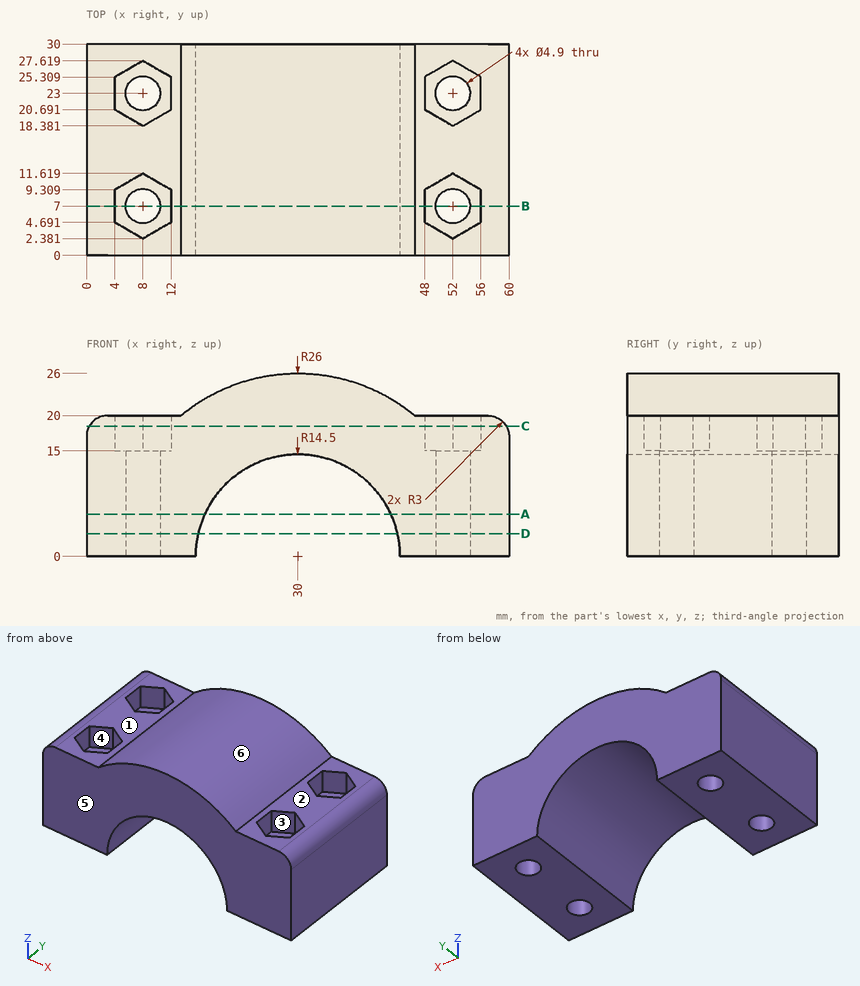
Design review of the part shown in the three views and the two pictorial views. Dimensions are in mm from the part's minimum x, y and z. A direction names the side the tool comes from. Round coordinates to 2 decimals unless told otherwise and drop trailing zeros. Write each loop counter-clockwise with the first axis right and the second up, starting at its lowest first coordinate (ties: lowest second). Pieces come first, ordered by that corner, then holes. Notation, with made-up numbers: (-15, 2) - (-8, 2) arc R28 ccw to (-8, 31) - close; hole circle Ø1 at (54.5, 51). An arc over 180 degrees is marked (long way). Answer as CSV lines item,"result". Start each with the question number.
(1) Add section A-A, the plane z = 6. State the section outline as (x, y) points.
(2) Add section D-D, the plane z = 3.25. State the section outline as (x, y) points.
(3) Mouldability with a two-part tool opening along Y and no side actions: class the marked faces 4, 5 and 6 as +Y half, -Y half, draft (parallel to the pull), parting line (faces both ways), or undercut.
(4) Add section B-B, the plane y = 7. State the section outline as (x, z) points.
(5) For pin 1 (4.5 mm diameter, centred on x = 8, y = 7, fed in from +Z); pin 2 (2 mm diameter, centred on x = 37, y = 4, fed in from +Z); pin 3 (4 mm diameter, centred on x = 7, y = 24, fed in from +Z); pin 4 (9 mm diameter, centred on x = 50, y = 7, fed in from +Z) (1 decimal), all flat-tipped, find the tip position at first contact; note any pin that passes through.
(6) For line 1 (Y direction, x = 52, z = 9.5); line 2 (X direction, y = 24.5, z = 3.5); line 3 (X direction, y = 7, z = 9.75), list the stretches that pass through material, from the lowest coordinate up.
(7) Add section C-C, the plane z = 18.5. State the section outline as (x, y) points.
(8) Machinability: for the marked faces 1, 2 and 3, which of the approach directions +Z, -Z, +X, -X, +Y, -Y give a long, thin tool a straight path to every point of the face, cutting with its end or side? Answer none if there is none.
From the geometry:
1,outline,"(0, 0) - (16.8, 0) - (16.8, 30) - (0, 30) - close; (43.2, 0) - (60, 0) - (60, 30) - (43.2, 30) - close; hole circle Ø4.9 at (8, 7); hole circle Ø4.9 at (8, 23); hole circle Ø4.9 at (52, 7); hole circle Ø4.9 at (52, 23)"
2,outline,"(0, 0) - (15.87, 0) - (15.87, 30) - (0, 30) - close; (44.13, 0) - (60, 0) - (60, 30) - (44.13, 30) - close; hole circle Ø4.9 at (8, 7); hole circle Ø4.9 at (8, 23); hole circle Ø4.9 at (52, 7); hole circle Ø4.9 at (52, 23)"
3,face 4,"undercut"
3,face 5,"-Y half"
3,face 6,"draft"
4,outline,"(0, 0) - (5.55, 0) - (5.55, 15) - (4, 15) - (4, 20) - (3, 20) arc R3 ccw to (0, 17) - close; (10.45, 0) - (15.5, 0) arc R14.5 cw to (44.5, 0) - (49.55, 0) - (49.55, 15) - (48, 15) - (48, 20) - (46.61, 20) arc R26 ccw to (13.39, 20) - (12, 20) - (12, 15) - (10.45, 15) - close; (54.45, 0) - (60, 0) - (60, 17) arc R3 ccw to (57, 20) - (56, 20) - (56, 15) - (54.45, 15) - close"
5,pin 1,"passes through"
5,pin 2,"stops at z = 25.3"
5,pin 3,"stops at z = 15"
5,pin 4,"stops at z = 20.9"
6,line 1,"y = 0 to 4.55, 9.45 to 20.55, 25.45 to 30"
6,line 2,"x = 0 to 6.06, 9.94 to 15.93, 44.07 to 50.06, 53.94 to 60"
6,line 3,"x = 0 to 5.55, 10.45 to 19.27, 40.73 to 49.55, 54.45 to 60"
7,outline,"(0.4, 0) - (59.6, 0) - (59.6, 30) - (0.4, 30) - close; hole (4, 4.69) - (8, 2.38) - (12, 4.69) - (12, 9.31) - (8, 11.62) - (4, 9.31) - close; hole (4, 20.69) - (8, 18.38) - (12, 20.69) - (12, 25.31) - (8, 27.62) - (4, 25.31) - close; hole (48, 4.69) - (52, 2.38) - (56, 4.69) - (56, 9.31) - (52, 11.62) - (48, 9.31) - close; hole (48, 20.69) - (52, 18.38) - (56, 20.69) - (56, 25.31) - (52, 27.62) - (48, 25.31) - close"
8,face 1,"+Z, -X, +Y, -Y"
8,face 2,"+Z, +X, +Y, -Y"
8,face 3,"+Z"
